Part model, mm, in its own coordinate system. Face numbers are marked on the shaded views. A direction names the side the tool comes from. Round coordinates to 2 decimals unless told otherwise and drop trailing zeros. Loops run counter-clockwise (first coordinate to the right, second up) from the corner with the lowest first, then second, coordinate; pieces in that order, holes last.
1) Probe line 1 (Y direction, x = -7, z = 0.5); line 2 (X direction, y = 4.5, z = -16.5); line 3 (X direction, y = 1, z = -13.5). List the from-to ranges inside material, lowest first.
2) Band-saw the part on C-C, the plane y = 1.5. Write the cut outline in (x, z).
3) Band-saw the part on B-B, the plane x = 0. Write the cut outline in (y, z).
4) Band-saw the part on A-A, the plane y = 11. Write the cut outline in (x, z).
5) 3-axis set-ups, long thin cutter, end or side, ignore diameter. For the marked faces 1, 2, 3, 4 and 5: which of +Z, -Z, +X, -X, +Y, -Y reach the whole face in a straight line?
6) Drop flat-ended pins along their axis: P1, Ø1.3, axis at x = -15.5, y = 8.5, coming from the -Z side; P2, Ø8, axis at x = 5.5, z = 9.5, coming from the +Y side; P3, Ø3.5, axis at x = 16, y = 9.5, coming from the +Z side. Give the stop position or say it passes through.
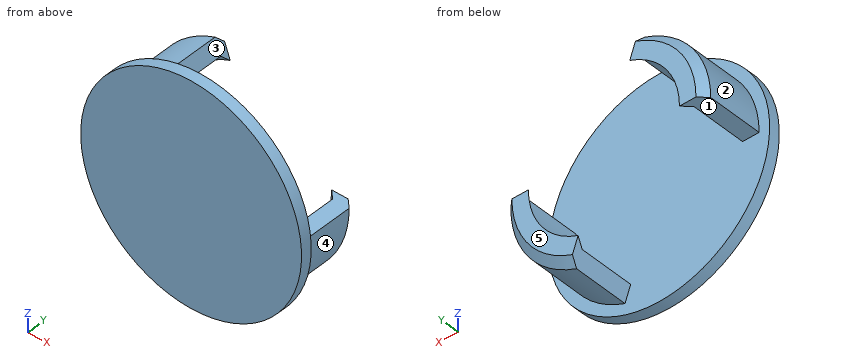
from build123d import *

# Parameters (mm, degrees)
SKETCH1_R           = 20
BOSS_EXTRUDE1_DEPTH = 2
REVOLVE1_ANGLE      = 70


with BuildPart() as part:
    # Sketch1 → Boss-Extrude1 (new body)
    with BuildSketch(Plane(origin=(0, 0, 0), x_dir=(1, 0, 0), z_dir=(0, 1, 0))):
        with Locations(Location((0, 0, 0), (0, 0, 270))):
            Circle(SKETCH1_R)
    extrude(amount=BOSS_EXTRUDE1_DEPTH)

    # Sketch2 → Revolve1 (revolve)
    with BuildSketch(Plane.XY):
        Polygon((18.1, 12), (16.669921141, 13.414213562), (13.685786438, 13.414213562), (15.1, 12), (15.1, 2), (18.1, 2), align=None)
        Polygon((-15.1, 2), (-15.1, 12), (-13.685786438, 13.414213562), (-16.669921141, 13.414213562), (-18.1, 12), (-18.1, 2), align=None)
    revolve(axis=Axis((0, 0, 0), (0, 1, 0)), revolution_arc=REVOLVE1_ANGLE)


solid = part.part
Reported:
1. line 1: y = 0 to 2
1. line 2: x = 6.01 to 7.44
1. line 3: x = -14.76 to 14.76
2. outline: circle Ø40 at (0, 0)
3. outline: (0, -20) - (2, -20) - (2, 20) - (0, 20) - close
4. outline: (-18.1, 0) - (-15.1, 0) arc R15.1 cw to (-5.16, 14.19) - (-6.19, 17.01) arc R18.1 ccw to start; (5.16, -14.19) - (6.19, -17.01) arc R18.1 ccw to (18.1, 0) - (15.1, 0) arc R15.1 cw to start
5. face 1: -Z, -X, +Y
5. face 2: +Z, -X, +Y
5. face 3: +Z, +X, +Y
5. face 4: -Z, +X, +Y
5. face 5: +Z, -Z, +X, -X, +Y
6. P1: stops at z = 0
6. P2: stops at y = 2
6. P3: stops at z = 0
